Part model, mm, in its own coordinate system. A direction names the side the tool comes from. Round coordinates to 2 decimals unless told otherwise and drop trailing zeros.
1) Drill centre lines: L1, parallel to Y at x = -5.5, z = -9.5; L2, parallel to Y at x = 4.5, z = -27. Where is each one in solid material? Low to high.
2) Pull direction Y, two halves, no side cores. Call faces 1 (the cylindrical face through (-2.71, -0.86, 0.59)), 2 (the flat face through (4, 7.5, 1)), 3 (the flat face through (6, 2, 1)), 4 (the flat face through (7.5, -4, 1)): +Y half, -Y half, draft (parallel to the pull), parting line (faces both ways), or undercut.
3) Which spindle directions (+Z, -Z, +X, -X, +Y, -Y) get a long thin tool onto all of the face, cutting with end or side? Do faces 5 (the flat face through (-2, 6, 1)), 6 (the flat face through (-2, -6, 1)), 7 (the flat face through (-6, -2, 1)), 8 (the flat face through (-2, 0, 42.5)). Say none if no direction does.
```python
from build123d import *

# Parameters (mm, degrees)
BOSS_EXTRUDE1_DEPTH = 42.5


with BuildPart() as part:
    # Sketch4 → Boss-Extrude1 (new body, symmetric)
    with BuildSketch(Plane.XY):
        with BuildLine():
            Line((2.4, -7.5), (6.1, -7.5))
            ThreePointArc((6.1, -7.5), (7.089949494, -7.089949494), (7.5, -6.1))
            Line((7.5, -6.1), (7.5, -2.4))
            ThreePointArc((7.5, -2.4), (7.382842712, -2.117157288), (7.1, -2))
            Line((7.1, -2), (5.595331881, -2))
            ThreePointArc((5.595331881, -2), (5.312489168, -2.117157288), (5.195331881, -2.4))
            Line((5.195331881, -2.4), (5.195331881, -2.6))
            ThreePointArc((5.195331881, -2.6), (4.948405254, -2.969551813), (4.512489168, -2.882842712))
            Line((4.512489168, -2.882842712), (3.202943725, -1.57329727))
            ThreePointArc((3.202943725, -1.57329727), (2.682689122, -0.794681232), (2.5, 0.123759005))
            Line((2.5, 0.123759005), (2.5, 0))
            Line((2.5, 0), (1.25, 0))
            ThreePointArc((1.25, 0), (0.883883476, -0.883883476), (0, -1.25))
            Line((0, -1.25), (0, -2.5))
            Line((0, -2.5), (-0.123759005, -2.5))
            ThreePointArc((-0.123759005, -2.5), (0.794681232, -2.682689122), (1.57329727, -3.202943725))
            Line((1.57329727, -3.202943725), (2.882842712, -4.512489168))
            ThreePointArc((2.882842712, -4.512489168), (2.969551813, -4.948405254), (2.6, -5.195331881))
            Line((2.6, -5.195331881), (2.4, -5.195331881))
            ThreePointArc((2.4, -5.195331881), (2.117157288, -5.312489168), (2, -5.595331881))
            Line((2, -5.595331881), (2, -7.1))
            ThreePointArc((2, -7.1), (2.117157288, -7.382842712), (2.4, -7.5))
        make_face()
    extrude(amount=BOSS_EXTRUDE1_DEPTH, both=True)

    # Mirror1: part across plane


with BuildPart() as part_1:
    add(part.part)
    add(part.part.mirror(Plane(origin=(0, 0, 0), x_dir=(0, 0, 1), z_dir=(1, 0, 0))))

    # Mirror2: part across plane


with BuildPart() as part_2:
    add(part_1.part)
    add(part_1.part.mirror(Plane.ZX))


solid = part_2.part
```
Completed:
1. L1: y = -7.5 to -2.01, 2.01 to 7.5
1. L2: y = -7.5 to -2.87, 2.87 to 7.5
2. face 1: undercut
2. face 2: +Y half
2. face 3: undercut
2. face 4: draft
3. face 5: +Z, -Z, +Y
3. face 6: +Z, -Z, -Y
3. face 7: +Z, -Z, -X
3. face 8: +Z, +X, -X, +Y, -Y
